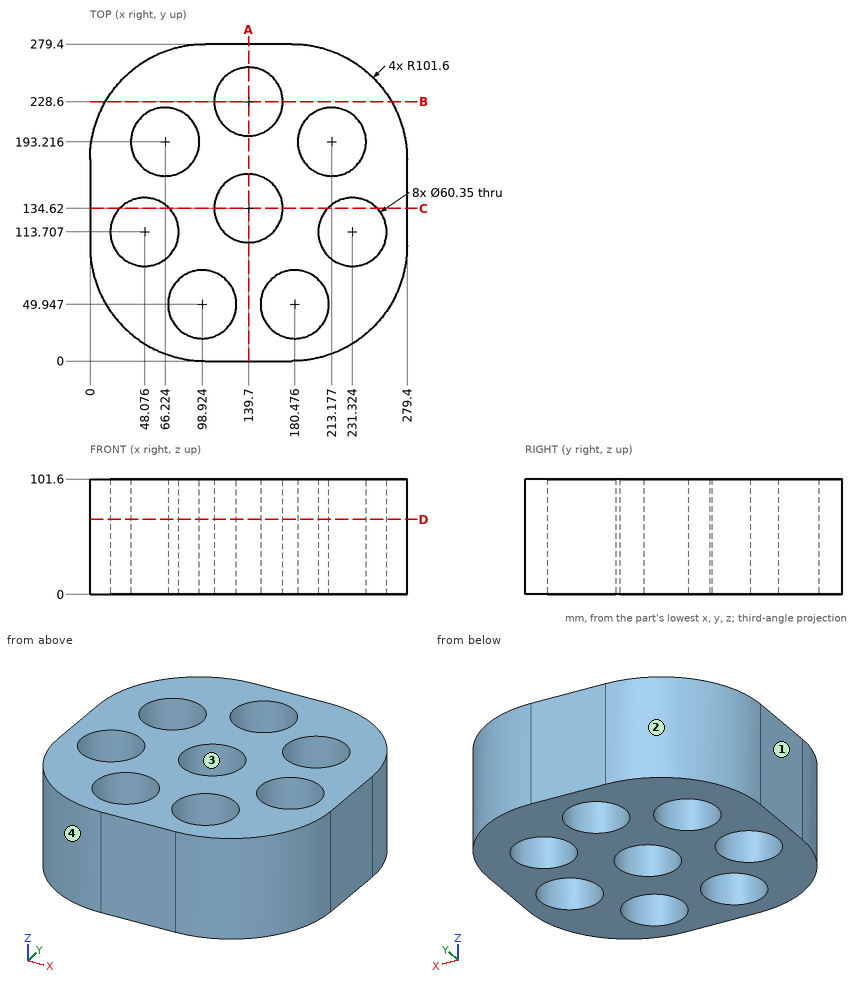
The drawing under review shows one solid part. Ordinate dimensions are in mm from its lowest x, y, z. Coordinates: 2 decimals unless noted, no trailing zeros. Write each loop counter-clockwise with the first axis right and the second up, starting at its lowest first coordinate (ties: lowest second). Pieces come first, ordered by that corner, then holes.
1) Insertion check: pin 1 (5 mm diameter, centred on x = 189.5, z = 81.5, fed in from +Y); pin 2 (5 mm diameter, centred on y = 246.5, z = 84, fed in from -X); pin 3 (1 mm diameter, centred on x = 60, z = 75.5, fed in from +Y) (1 decimal). Each pin has a flat end and moves straight along its axis. Give the tip position at first contact, or say it passes through.
2) Add section C-C (y = 134.62). Write out the cut boundary in (x, z) (1 decimal), plus the area to 3 significant figures.
3) Add section B-B (y = 228.6). Write out the cut boundary in (x, z) (1 decimal).
4) Mouldability with a two-part tool opening along Y and no side actions: class the marked faces 1, 2, 3 and 4 as +Y half, -Y half, draft (parallel to the pull), parting line (faces both ways), or undercut.
5) To check wall thickness, follow L1, parallel to Y at x = 139.7, z = 48.5 (1 decimal); L2, parallel to X at y = 102, z = 66.5 (1 decimal); L3, parallel to X at y = 116.5, z = 23.5. State the ranges of each line that lie inside material, in increasing order.
6) Add section A-A (x = 139.7). Write out the cut boundary in (y, z) (1 decimal), plus the area to 3 significant figures.
7) Add section D-D (z = 66). State how many separate pieces and enclosed holes the cut face has, plus the area to 3 significant figures.
Check result:
1. pin 1: stops at y = 278.98
1. pin 2: stops at x = 24.53
1. pin 3: stops at y = 270.7
2. outline: (0, 0) - (26.3, 0) - (26.3, 101.6) - (0, 101.6) - close; (69.8, 0) - (109.5, 0) - (109.5, 101.6) - (69.8, 101.6) - close; (169.9, 0) - (209.6, 0) - (209.6, 101.6) - (169.9, 101.6) - close; (253.1, 0) - (279.4, 0) - (279.4, 101.6) - (253.1, 101.6) - close
2. area: 13,400 mm2
3. outline: (13.6, 0) - (109.5, 0) - (109.5, 101.6) - (13.6, 101.6) - close; (169.9, 0) - (265.8, 0) - (265.8, 101.6) - (169.9, 101.6) - close
4. face 1: draft
4. face 2: +Y half
4. face 3: undercut
4. face 4: -Y half
5. L1: y = 0 to 104.4, 164.8 to 198.4, 258.8 to 279.4
5. L2: x = 0 to 20.3, 75.9 to 203.5, 259.1 to 279.4
5. L3: x = 0 to 18.03, 78.12 to 115.57, 163.83 to 201.28, 261.37 to 279.4
6. outline: (0, 0) - (104.4, 0) - (104.4, 101.6) - (0, 101.6) - close; (164.8, 0) - (198.4, 0) - (198.4, 101.6) - (164.8, 101.6) - close; (258.8, 0) - (279.4, 0) - (279.4, 101.6) - (258.8, 101.6) - close
6. area: 16,100 mm2
7. separate pieces: 1
7. enclosed holes: 8
7. area: 46,300 mm2
